```python
from build123d import *

# Parameters (mm, degrees)
F0_W = 21.49
F0_H = 3.925


with BuildPart() as f1:
    # F0 (on Right) → F1 (revolve)
    with BuildSketch(Plane.YZ):
        Polygon((0, 5.675), (0, 0), (0.33, 0), (0.33, 6.005), align=None)
        Polygon((0.33, 6.005), (0.33, 0), (1.24, 0), (2.08, 0), (2.08, 5.195), (1.24, 5.195), (1.24, 6.005), align=None)
        Polygon((2.08, 5.195), (2.08, 0), (3.16, 0), (3.16, 5.98), align=None)
        Polygon((3.16, 5.98), (3.16, 0), (49.49, 0), (49.49, 5.6), align=None)
        Polygon((49.49, 5.6), (49.49, 0), (53.56, 0), (63.35, 0), (63.35, 3.925), (63.35, 4.3153), (53.56, 4.3153), align=None)
        with Locations((74.095, 1.9625)):
            Rectangle(F0_W, F0_H)
    revolve(axis=Axis((0, 26.325, 0), (0, 1, 0)))


solid = f1.part
```
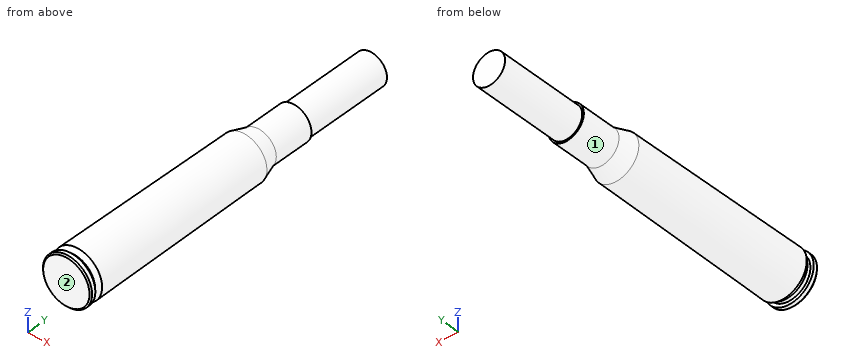
Can you work these out from the model? Positions are in its coordinate system, mm. Face numbers are marked on the shaded views. A direction names the side the tool comes from. Round coordinates to 2 decimals unless told otherwise and drop trailing zeros. Loops run counter-clockwise (first coordinate to the right, second up) from the corner with the lowest first, then second, coordinate; pieces in that order, holes last.
Item 1: Suppose I cut it at A-A, the plane y = 48.5. Write out the boundary of the cut face in (x, z).
Item 2: Suppose I cut it at B-B, the plane y = 28. Write out the boundary of the cut face in (x, z).
Item 3: Which directions (+Z, -Z, +X, -X, +Y, -Y) give clear straight access to the entire face, cutting with the end or side of a thin tool? Please do the marked faces 1 and 2.
Item 4: Please list where these lines run through material, in increasing order: L1, parallel to X at y = 15, z = 2.75; L2, parallel to X at y = 12, z = -4.25; L3, parallel to Z at x = -0.5, y = 65.
Item 5: Will these pins go through, and if not, where does the flat tip stop? pin 1 Ø4 at (x, y) = (-0.5, 18.5) entering from +Z; pin 2 Ø2 at (y, z) = (21.5, 2) entering from +X; pin 3 Ø4 at (y, z) = (75, 2.5) entering from -X.
Reported:
1. outline: circle Ø11.22 at (0, 0)
2. outline: circle Ø11.55 at (0, 0)
3. face 1: +Y
3. face 2: +Z, -Z, +X, -X, -Y
4. L1: x = -5.2 to 5.2
4. L2: x = -4.1 to 4.1
4. L3: z = -3.89 to 3.89
5. pin 1: stops at z = 5.87
5. pin 2: stops at x = 5.74
5. pin 3: stops at x = -3.89
